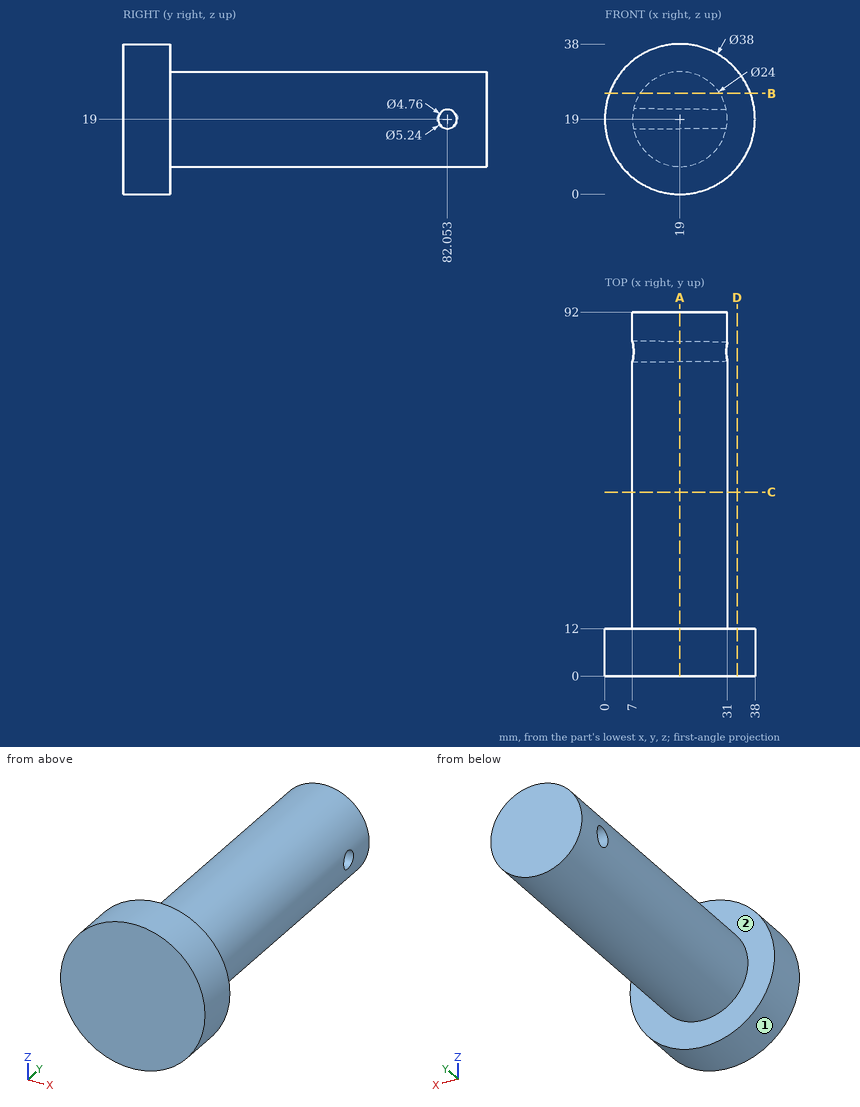
Geometry: see drawing. Coordinates: mm, zero at the bounding-box minimum. A direction names the side the tool comes from. Round coordinates to 2 decimals unless told otherwise and drop trailing zeros. Loops run counter-clockwise (first coordinate to the right, second up) from the corner with the lowest first, then second, coordinate; pieces in that order, holes last. Notation, with made-up numbers: (-10, -29.5) - (42, -29.5) arc R30 cw to (42, -3.5) - close; hole circle Ø8 at (53, 83.25). An arc over 180 degrees is marked (long way). Use CSV: the item, a comma, the result in double quotes.
Q1. Section query C-C, the plane y = 46.5. Output: boundary loops of the cut face in (x, z).
Reported:
outline,"circle Ø24 at (19, 19)"
Q2. Section query A-A, the plane x = 19. Output: boundary loops of the cut face in (y, z).
Reported:
outline,"(0, 0) - (12, 0) - (12, 7) - (92, 7) - (92, 31) - (12, 31) - (12, 38) - (0, 38) - close; hole circle Ø5 at (82.05, 19)"
Q3. Pin query (flat end, axial travel): pin 1 Ø1.5 at (x, z) = (10, 27) entering from +Y; pin 2 Ø10 at (x, y) = (22.5, 19) entering from +Z; pin 3 Ø10 at (x, y) = (18.5, 35) entering from -Z; pin 4 Ø1 at (x, y) = (32, 57.5) entering from -Z. Return the tip coordinate at first contact, or that it passes through.
Reported:
pin 1,"y = 92"
pin 2,"z = 31"
pin 3,"z = 7"
pin 4,"through"
Q4. Section query B-B, the plane z = 25.5. Output: boundary loops of the cut face in (x, y).
Reported:
outline,"(1.15, 0) - (36.85, 0) - (36.85, 12) - (29.09, 12) - (29.09, 92) - (8.91, 92) - (8.91, 12) - (1.15, 12) - close"
Q5. Reachability of the marked faces 1 and 2 from +Z, -Z, +X, -X, +Y, -Y: full face, straight path, thin tool, end or side. Return the list, or none.
Reported:
face 1,"+Y, -Y"
face 2,"+Y"
Q6. Ray query, line 1 along Y through (x, z) = (34.5, 15.5); line 2 along X through (y, z) = (41.5, 18.5); line 3 along Y through (x, z) = (30, 18) (1 decimal). Return the intervals inside material, ascending.
Reported:
line 1,"0 to 12"
line 2,"7.01 to 30.99"
line 3,"0 to 79.9, 84.2 to 92"
Q7. Section query D-D, the plane x = 33.5. Output: boundary loops of the cut face in (y, z).
Reported:
outline,"(0, 6.72) - (12, 6.72) - (12, 31.28) - (0, 31.28) - close"
